Part model, mm, in its own coordinate system. Round coordinates to 2 decimals unless told otherwise and drop trailing zeros. Write each loop counter-clockwise with the first axis right and the second up, starting at its lowest first coordinate (ties: lowest second). Pieces come first, ordered by that corner, then holes. Notation, with made-up numbers: M 83,-8.5 L 92,-8.5 A20 ccw 92,15.5 Z; hole C -37.5,86.25 d8. An arc over 180 degrees is marked long. Answer as a JSON object with one key per item and string values. Group by question number.
1. Drill centre lines: line 1 (Y direction, x = 35, z = 3.7); line 2 (X direction, y = 1.5, z = 5); line 3 (Y direction, x = -54.5, z = 5.15). Where is each one in solid material? Low to high. Write a range as from..to.
2. Band-saw the part on C-C, the plane z = 4. Count the separate pieces of the cut face and the enclosed holes in it, plus the area to 3 significant figures.
3. Drop flat-ended pins along their axis: pin 1 (1.6 mm diameter, centred on x = -55, z = 4, fed in from +Y); pin 2 (3 mm diameter, centred on y = -90, z = 2, fed in from -X). Give the stop position or say it passes through.
4. Band-saw the part on A-A, the plane x = 35. Write the cut outline in (y, z), plus the area to 3 significant figures.
5. Band-saw the part on D-D, the plane x = -34.5. Write the cut outline in (y, z).
6. Band-saw the part on B-B, the plane y = -31.5. Write the cut outline in (x, z), plus the area to 3 significant figures.
Autodesk Inventor part; units mm, degrees
ref_plane "YZ Plane" through (0, 0, 0) normal (1, 0, 0) x (0, 1, 0)
ref_plane "XZ Plane" through (0, 0, 0) normal (0, 1, 0) x (-1, 0, 0)
ref_plane "XY Plane" through (0, 0, 0) normal (0, 0, 1) x (1, 0, 0)
sketch "Sketch1" plane through (0, 0, 0) normal (0, 0, 1) x (1, 0, 0)
  line L0 (-20, 6) -> (-10, 6)
  line L1 (-70, 0) -> (-70, 6)
  line L2 (-75, 6) -> (-70, 6)
  line L3 (-75, 0) -> (-75, 6)
  line L4 (-75, 0) -> (-70, 0)
  line L5 (40, -67) -> (40, -9)
  line L6 (40, 6) -> (-75, 6)
  line L7 (-75, 6) -> (-75, -94)
  line L8 (-75, -94) -> (40, -94)
  line L9 (40, -94) -> (40, 6)
  dimension "d85" = 115
  dimension "d86" = 100
extrude "Extrusion1" add sketch "Sketch1" along normal blind 6 contours L0 L6 L9 L5 L8 L7 L4 L1
ref_plane "Work Plane1" through (-75, -44, 0) normal (0, -1, 0) x (1, 0, 0)
sketch "Sketch2" plane through (0, 0, 6) normal (0, 0, 1) x (1, 0, 0)
  line L0 (-60, 6) -> (-60, 0)
  line L1 (-60, 0) -> (-50, 0)
  line L2 (-50, 0) -> (-50, 6)
  line L3 (-40, 0) -> (-30, 0)
  line L4 (-30, 0) -> (-30, 6)
  line L5 (-40, 6) -> (-40, 0)
  line L6 (-20, 0) -> (-10, 0)
  line L7 (-20, 6) -> (-20, 0)
  line L8 (-10, 0) -> (-10, 6)
  line L9 (40, 6) -> (-70, 6)
  line L10 (-50, 6) -> (-49.9, 6)
  line L11 (-49.9, 6) -> (-49.9, 0)
  line L12 (-49.9, 0) -> (-50, 0)
  line L13 (-50, 0) -> (-50, 6)
  line L14 (-60, 6) -> (-60.1, 6)
  line L15 (-60.1, 6) -> (-60.1, 0)
  line L16 (-60.1, 0) -> (-60, 0)
  line L17 (-60, 0) -> (-60, 6)
  point P0 (0, 0)
  dimension "d5" = 0.1
  dimension "d6" = 6
  dimension "d7" = 0.1
  dimension "d8" = 6
extrude "Extrusion2" cut sketch "Sketch2" against normal blind 6 contours L9 L2 L1 L0 | L0 L16 L15 L9 | L9 L11 L12 L2
pattern_linear "Rectangular Pattern1" count 3 spacing 20 along (1, 0, 0) of "Extrusion2"
sketch "Sketch3" plane through (0, 0, 6) normal (0, 0, 1) x (1, 0, 0)
  circle A0 centre (35, -76.5) radius 1.6
  line L0 (-90, -94) -> (40, -94)
  line L1 (40, -94) -> (40, 6)
  circle A1 centre (35, -61.5) radius 1.6
  circle A2 centre (35, -46.5) radius 1.6
  circle A3 centre (35, -31.5) radius 1.6
  circle A4 centre (35, -16.5) radius 1.6
  point P0 (0, 0)
  point P1 (35, -59)
  point P2 (35, -39)
  point P3 (35, -29)
  point P4 (35, -49)
  point P5 (35, -19)
  dimension "d73" = 3.2
  dimension "d74" = 17.5
  dimension "d75" = 5
  dimension "d78" = 15
sketch "Sketch4" plane through (0, 0, 6) normal (0, 0, 1) x (1, 0, 0)
  line L0 (-60.1, 0) -> (-60.1, 6)
  line L1 (-60, 0) -> (-50, 0)
  line L2 (-49.9, 6) -> (-49.9, 0)
  line L3 (-49.9, 0) -> (-60.1, 0)
  line L4 (66, -44) -> (-116, -44)
  line L5 (-60.1, -88) -> (-60.1, -94)
  line L6 (-49.9, -94) -> (-49.9, -88)
  line L7 (-49.9, -88) -> (-60.1, -88)
  line L8 (-90, -94) -> (40, -94)
  line L9 (-69.9, -94) -> (-69.9, -88)
  line L10 (-69.9, -88) -> (-80.1, -88)
  line L11 (-80.1, -88) -> (-80.1, -94)
  line L12 (-29.9, -94) -> (-29.9, -88)
  line L13 (-29.9, -88) -> (-40.1, -88)
  line L14 (-40.1, -88) -> (-40.1, -94)
  line L15 (-49.9, -94) -> (-49.9, -88)
  line L16 (-49.9, -88) -> (-60.1, -88)
  line L17 (-60.1, -88) -> (-60.1, -94)
  line L18 (-9.9, -94) -> (-9.9, -88)
  line L19 (-9.9, -88) -> (-20.1, -88)
  line L20 (-20.1, -88) -> (-20.1, -94)
  line L21 (-29.9, -94) -> (-29.9, -88)
  line L22 (-29.9, -88) -> (-40.1, -88)
  line L23 (-40.1, -88) -> (-40.1, -94)
  line L24 (10.1, -94) -> (10.1, -88)
  line L25 (10.1, -88) -> (-0.1, -88)
  line L26 (-0.1, -88) -> (-0.1, -94)
  line L27 (-9.9, -94) -> (-9.9, -88)
  line L28 (-9.9, -88) -> (-20.1, -88)
  line L29 (-20.1, -88) -> (-20.1, -94)
  line L30 (30.1, -94) -> (30.1, -88)
  line L31 (30.1, -88) -> (19.9, -88)
  line L32 (19.9, -88) -> (19.9, -94)
  line L33 (10.1, -94) -> (10.1, -88)
  line L34 (10.1, -88) -> (-0.1, -88)
  line L35 (-0.1, -88) -> (-0.1, -94)
  point P0 (0, 0)
  point P1 (19.9, -94)
  point P2 (30.1, -94)
  point P3 (-0.1, -94)
  point P4 (10.1, -94)
  point P5 (-20.1, -94)
  point P6 (-9.9, -94)
  point P7 (-40.1, -94)
  point P8 (-29.9, -94)
  point P9 (-80.1, -94)
  point P10 (-69.9, -94)
  dimension "d16" = 20
  dimension "d19" = 20
extrude "Extrusion4" cut sketch "Sketch4" against normal blind 6
sketch "Sketch6" plane through (0, 0, 6) normal (0, 0, 1) x (1, 0, 0)
  line L0 (-69.9, -88) -> (-75, -88)
  line L1 (-75, -88) -> (-74.8, -88)
  line L2 (-74.8, -88) -> (-74.8, -86)
  line L3 (-74.8, -86) -> (-75, -86)
  line L4 (-75, -86) -> (-75, -88)
  line L5 (-75, -88) -> (-75.2, -88)
  line L6 (-75.2, -88) -> (-75.2, -86)
  line L7 (-75.2, -86) -> (-75, -86)
  line L8 (-75, -86) -> (-75, -88)
  point P0 (0, 0)
  point P1 (-80.1, -88)
  dimension "d40" = 0.2
  dimension "d41" = 2
  dimension "d42" = 0.2
  dimension "d43" = 2
extrude "Extrusion6" cut sketch "Sketch6" against normal blind 0.2
sketch "Sketch7" plane through (0, 0, 6) normal (0, 0, 1) x (1, 0, 0)
  line L0 (27.75, -85) -> (22.25, -85)
  line L1 (22.25, -85) -> (22.25, -82.6)
  line L2 (22.25, -82.6) -> (27.75, -82.6)
  line L3 (27.75, -82.6) -> (27.75, -85)
  line L4 (10.1, -94) -> (19.9, -94)
  line L5 (30.1, -88) -> (30.1, -94)
  line L6 (-57.75, -82.6) -> (-52.25, -82.6)
  line L7 (-52.25, -82.6) -> (-52.25, -85)
  line L8 (-52.25, -85) -> (-57.75, -85)
  line L9 (-57.75, -85) -> (-57.75, -82.6)
  line L10 (-12.25, -5.4) -> (-17.75, -5.4)
  line L11 (-17.75, -5.4) -> (-17.75, -3)
  line L12 (-17.75, -3) -> (-12.25, -3)
  line L13 (-12.25, -3) -> (-12.25, -5.4)
  line L14 (-20.1, 6) -> (-29.9, 6)
  line L15 (-9.9, 6) -> (-9.9, 0)
  line L16 (-52.25, -5.4) -> (-57.75, -5.4)
  line L17 (-57.75, -3) -> (-52.25, -3)
  line L18 (-52.25, -3) -> (-52.25, -5.4)
  line L19 (-57.75, -5.4) -> (-57.75, -3)
  point P0 (0, 0)
  dimension "d4" = 0
  dimension "d49" = 5.5
  dimension "d50" = 2.4
  dimension "d51" = 9
  dimension "d52" = 2.35
  dimension "d55" = 80
  dimension "d60" = 5.5
  dimension "d61" = 2.4
  dimension "d62" = 9
  dimension "d63" = 2.35
  dimension "d66" = 40
extrude "Extrusion7" cut sketch "Sketch7" against normal blind 6
extrude "Extrusion8" cut sketch "Sketch3" against normal through all
properties part number "00_Baseplate_Simmo_side2_v2"
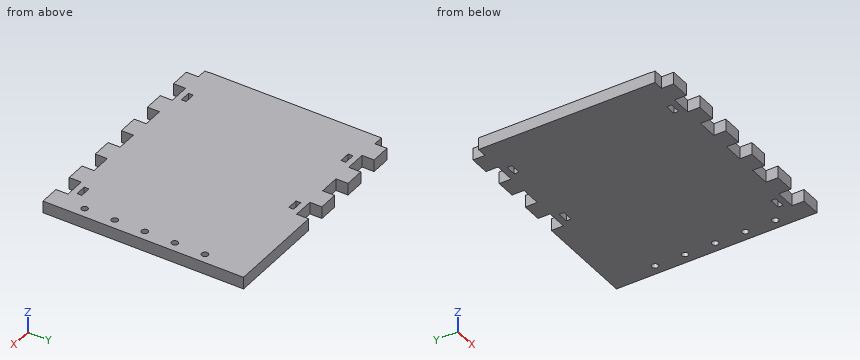
Worked answers:
{
 "1": {"line 1": "y = -94..-78.1, -74.9..-63.1, -59.9..-48.1, -44.9..-33.1, -29.9..-18.1, -14.9..6", "line 2": "x = -70..-60.1, -49.9..-40.1, -29.9..-20.1, -9.9..40", "line 3": "y = -88..-85, -82.6..-5.4, -3..0"},
 "2": {"separate pieces": "1", "enclosed holes": "9", "area": "10,900 mm^2"},
 "3": {"pin 1": "stops at y = 0", "pin 2": "stops at x = -69.9"},
 "4": {"outline": "M -94,0 L -78.1,0 L -78.1,6 L -94,6 Z; M -74.9,0 L -63.1,0 L -63.1,6 L -74.9,6 Z; M -59.9,0 L -48.1,0 L -48.1,6 L -59.9,6 Z; M -44.9,0 L -33.1,0 L -33.1,6 L -44.9,6 Z; M -29.9,0 L -18.1,0 L -18.1,6 L -29.9,6 Z; M -14.9,0 L 6,0 L 6,6 L -14.9,6 Z", "area": "504 mm^2"},
 "5": {"outline": "M -88,0 L 0,0 L 0,6 L -88,6 Z"},
 "6": {"outline": "M -75,0 L 33.4,0 L 33.4,6 L -75,6 Z; M 36.6,0 L 40,0 L 40,6 L 36.6,6 Z", "area": "671 mm^2"}
}
